Build history of the part. All positions in model axes, mm. A direction names the side the tool comes from. Round coordinates to 2 decimals unless told otherwise and drop trailing zeros. Order: outer loops, then holes, each group sorted by start corner. A loop starts at its lowest first (then second) coordinate and runs counter-clockwise, first axis right, second up. Notation, with made-up numbers: M 43.5,5.25 L 92.5,5.25 A16 ccw 92.5,33.25 Z; hole C 67.5,61.5 d8. An arc over 180 degrees is marked long. One line per item, written item: value. Start each with the question number.
Item 1: Probe L1, parallel to Y at x = 12.5, z = 0; L2, parallel to Z at x = 7.5, y = -0.5; L3, parallel to X at y = -25.5, z = -27. List the from-to ranges inside material, lowest first.
Item 2: Band-saw the part on C-C, the plane x = 6.5. Write the cut outline in (y, z), then the cut area to 3 significant figures.
Item 3: Pin check, flat tips, straight feed: pin 1 (1.5 mm diameter, centred on x = 7, z = 3, fed in from +Y); pin 2 (12 mm diameter, centred on x = 25, y = -26, fed in from +Z); pin 3 (16 mm diameter, centred on y = 55, z = 0, fed in from +X); pin 4 (5 mm diameter, centred on x = 21, y = 17.5, fed in from -Z). Stop position of each tip, or through.
Item 4: Band-saw the part on A-A, the plane z = 0. Give the number of separate pieces and of enclosed holes in the cut face, then the cut area to 3 significant figures.
Item 5: Band-saw the part on B-B, the plane y = -55. Write the cut outline in (x, z), then the cut area to 3 significant figures.
Item 6: Tool access for faces 1 (the flat face through (3, -32, 32)), 2 (the cylindrical face through (10.395, -9.764, -74.362)), 3 (the flat face through (18, 34, 16)): list every direction of +Z, -Z, +X, -X, +Y, -Y with a clear straight run to the whole face (end or side of a thin tool).
Item 7: Two-plate mould, pull along Z, no slides. Class faces 4 (the flat face through (0, -19, 19)), 5 (the cylindrical face through (1.521, -42.954, -9.538)), 6 (the cylindrical face through (16.77, 23.21, -3.05)): +Z half, -Z half, draft (parallel to the pull), parting line (faces both ways), or undercut.
```python
from build123d import *

# Parameters (mm, degrees)
SKETCH1_W                      = 15
SKETCH1_H                      = 75
SKETCH2_R                      = 44
BOSS_EXTRUDE1_DEPTH            = 3
SKETCH3_R                      = 35
BOSS_EXTRUDE2_DEPTH            = 16
BOSS_EXTRUDE2_TAPER            = 4.57392126
F_18_0_18_DIAMETER_HOLE1_D     = 18
F_18_0_18_DIAMETER_HOLE1_DEPTH = 31
M42_CLEARANCE_HOLE1_D          = 46.820907
M42_CLEARANCE_HOLE1_DEPTH      = 34
CHAMFER1_SIZE                  = 0.7395465
FILLET1_R                      = 2.415


with BuildPart() as part:
    # Sketch1 → Revolve1 (revolve)
    with BuildSketch(Plane(origin=(0, 0, 0), x_dir=(-1, 0, 0), z_dir=(0, 0, -1))):
        with Locations((-10.5, 37.5)):
            Rectangle(SKETCH1_W, SKETCH1_H)
    revolve(axis=Axis((18, 0, 0), (-1, 0, 0)))

    # Sketch2 → Boss-Extrude1 (add)
    with BuildSketch(Plane.ZY.offset(-3)):
        Circle(SKETCH2_R)
    extrude(amount=BOSS_EXTRUDE1_DEPTH)

    # Sketch3 → Boss-Extrude2 (add)
    with BuildSketch(Plane(origin=(18, 0, 0), x_dir=(0, 0, -1), z_dir=(1, 0, 0))):
        Circle(SKETCH3_R)
    extrude(amount=BOSS_EXTRUDE2_DEPTH, taper=BOSS_EXTRUDE2_TAPER)

    # Ø18.0 (18) Diameter Hole1
    with Locations(Plane.ZY.offset(-3)):
        with Locations((0, -55), (-55, 0), (0, 55), (55, 0)):
            Hole(F_18_0_18_DIAMETER_HOLE1_D / 2, depth=F_18_0_18_DIAMETER_HOLE1_DEPTH)

    # M42 Clearance Hole1
    with Locations(Plane(origin=(34, 0, 0), x_dir=(0, 0, -1), z_dir=(1, 0, 0))):
        with Locations((0, 0)):
            Hole(M42_CLEARANCE_HOLE1_D / 2, depth=M42_CLEARANCE_HOLE1_DEPTH)

    # Chamfer1
    chamfer1_edges = [part.edges().sort_by_distance(p)[0] for p in [
        (34, 0, -23.4104535),
        (0, 0, -23.4104535),
    ]]
    chamfer(chamfer1_edges, length=CHAMFER1_SIZE)

    # Fillet1
    fillet1_edges = [part.edges().sort_by_distance(p)[0] for p in [
        (18, 0, 35),
    ]]
    fillet(fillet1_edges, radius=FILLET1_R)


solid = part.part
```
Output:
1. L1: y = -75 to -64, -46 to -23.41, 23.41 to 46, 64 to 75
1. L2: z = -75 to -63.99, -46.01 to -23.41, 23.41 to 46.01, 63.99 to 75
1. L3: x = 0 to 18
2. outline: C 0,0 d150; hole C -55,0 d18; hole C 0,0 d46.82; hole C 0,-55 d18; hole C 0,55 d18; hole C 55,0 d18
2. area: 14,900 mm²
3. pin 1: stops at y = 74.97
3. pin 2: stops at z = 28.08
3. pin 3: passes through
3. pin 4: stops at z = -31.46
4. separate pieces: 4
4. enclosed holes: 0
4. area: 1,480 mm²
5. outline: M 3,-50.99 L 18,-50.99 L 18,-9 L 3,-9 Z; M 3,9 L 18,9 L 18,50.99 L 3,50.99 Z
5. area: 1,260 mm²
6. face 1: -X
6. face 2: +X, -X
6. face 3: +X
7. face 4: draft
7. face 5: parting line
7. face 6: undercut
